Input: dimensioned drawing with shaded views. Units: mm. Origin: part minimum x, y, z. A direction names the side the tool comes from. Give positions to 0.01 mm unless a question says otherwise; leave off trailing zeros. Loops run counter-clockwise (first coordinate to the right, second up) from the corner with the lowest first, then second, coordinate; pieces in that order, holes last. Notation, with made-up numbers: (29, 70.25) -> (84, 70.25) arc R26 cw to (84, 103.25) -> close; hole circle Ø11 at (7.25, 38). An arc over 180 degrees is marked (long way). One line per question, with ' | ' between items. Start each with the question number.
Item 1: Section A-A on y = 19. Return loops of the section in (x, z).
Item 2: Mould query, pull axis Z, two halves, no side actions, for the marked faces 1, 2, 3 and 4. Classes: released by +Z, released by -Z, zero draft, split by the parting line, or undercut.
Item 3: Section D-D on z = 18. Return loops of the section in (x, y).
Item 4: Material intervals for line 1 along Z through (x, y) = (20.25, 59.5); line 2 along Y through (x, z) = (1.75, 84); line 3 along Z through (x, y) = (2.25, 17), sorted ascending. Write a range as [from, to].
Item 5: Section B-B on x = 18.5. Return loops of the section in (y, z).
Item 6: Pin query (flat end, axial travel): P1, Ø4, axis at x = 2.5, y = 43, coming from the -Z side; P2, Ø8, axis at x = 12, z = 64, coming from the +Y side. Return the tip coordinate at first contact, or that it passes through.
Item 7: Section C-C on y = 43. Return loops of the section in (x, z), then the cut area to 3 significant figures.
Item 8: Set-up query: the marked faces 5 and 6. Return all of +Z, -Z, +X, -X, +Y, -Y with unobstructed straight access to the full face (end or side cutting, diameter ignored); none if empty.
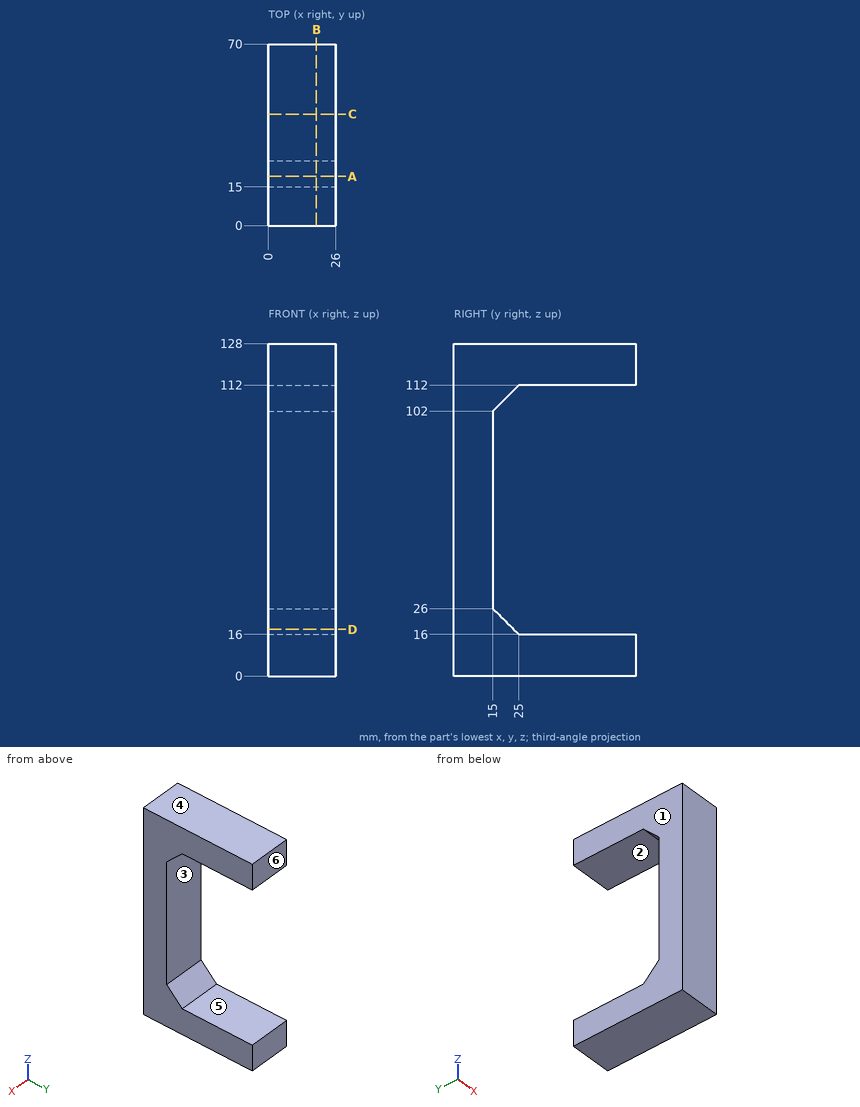
Result sheet:
1) outline: (0, 0) -> (26, 0) -> (26, 22) -> (0, 22) -> close; (0, 106) -> (26, 106) -> (26, 128) -> (0, 128) -> close
2) face 1: zero draft | face 2: undercut | face 3: undercut | face 4: released by +Z
3) outline: (0, 0) -> (26, 0) -> (26, 23) -> (0, 23) -> close
4) line 1: z = [0, 16], [112, 128] | line 2: y = [0, 15] | line 3: z = [0, 24], [104, 128]
5) outline: (0, 0) -> (70, 0) -> (70, 16) -> (25, 16) -> (15, 26) -> (15, 102) -> (25, 112) -> (70, 112) -> (70, 128) -> (0, 128) -> close
6) P1: stops at z = 0 | P2: stops at y = 15
7) outline: (0, 0) -> (26, 0) -> (26, 16) -> (0, 16) -> close; (0, 112) -> (26, 112) -> (26, 128) -> (0, 128) -> close | area: 832 mm²
8) face 5: +X, -X, +Y | face 6: +Z, -Z, +X, -X, +Y
